from build123d import *

# Parameters (mm, degrees)
CROQUIS1_R              = 1.5
SALIENTE_EXTRUIR1_DEPTH = 1
CORTAR_EXTRUIR1_DEPTH   = 1


with BuildPart() as part:
    # Croquis1 → Saliente-Extruir1 (new body)
    with BuildSketch(Plane(origin=(0, 0, 0), x_dir=(1, 0, 0), z_dir=(0, 1, 0))):
        Polygon((-3, 3), (-3, -49.8), (3, -49.8), (3, -43.8), (29, -26.4), (35, -26.4), (35, -20.4), (29, -20.4), (3, -3), (3, 3), align=None)
        with Locations(Location((0, 0, 0), (0, 0, 270))):
            Circle(CROQUIS1_R, mode=Mode.SUBTRACT)
        with Locations(Location((0, -46.8, 0), (0, 0, 270))):
            Circle(CROQUIS1_R, mode=Mode.SUBTRACT)
        with Locations(Location((32, -23.4, 0), (0, 0, 270))):
            Circle(CROQUIS1_R, mode=Mode.SUBTRACT)
    extrude(amount=SALIENTE_EXTRUIR1_DEPTH)

    # Croquis2 → Cortar-Extruir1 (cut)
    with BuildSketch(Plane(origin=(0, 4, 0), x_dir=(1, 0, 0), z_dir=(0, 1, 0))):
        Polygon((29, -20.4), (29, -26.4), (1.37887203, -65.195749652), (-23.269516781, -18.416533666), (-7.63010581, 16.328115394), align=None)
    extrude(amount=-CORTAR_EXTRUIR1_DEPTH, mode=Mode.SUBTRACT)


solid = part.part
Part model, mm, in its own coordinate system. A direction names the side the tool comes from. Coordinates: 2 decimals unless noted, no trailing zeros. Order: outer loops, then holes, each group sorted by start corner. A loop starts at its lowest first (then second) coordinate and runs counter-clockwise, first axis right, second up. Notation, with made-up numbers: M 8,86 L 12,86 A12 ccw 12,104 Z; hole C 68,73 d7. An arc over 180 degrees is marked long. One line per question, with ' | ' between items.
Q1. 3-axis set-ups, long thin cutter, end or side, ignore diameter. For faces 4 (the face through (0.45, 0.49, 1.43)), 5 (the face through (3, 0.5, 46.8)), 6 (the face through (32, 0.5, 20.4)): which of +Z, -Z, +X, -X, +Y, -Y reach the whole face in a straight line?
A:
face 4: +Y, -Y | face 5: +Z, +X, +Y, -Y | face 6: -Z, +X, +Y, -Y
Q2. Pin check, flat tip, straight feed: P1, Ø0.5, axis at x = 31, y = 0.5, coming from the +Z side. Stop position of the tip, or through.
A:
P1: stops at z = 26.4
Q3. Drill centre lines: line 1 (Z direction, x = 1, y = 0.6); line 2 (X direction, y = 0.7, z = 46.8); line 3 (X direction, y = 0.25, z = 23.4). Where is each one in solid material? Low to high.
A:
line 1: z = -3 to -1.12, 1.12 to 45.68, 47.92 to 49.8 | line 2: x = -3 to -1.5, 1.5 to 3 | line 3: x = -3 to 30.5, 33.5 to 35
Q4. Slice it at C-C (x = 0). Give the cut face in (y, z), and give its area (3 significant figures).
A:
outline: M 0,-3 L 1,-3 L 1,-1.5 L 0,-1.5 Z; M 0,1.5 L 1,1.5 L 1,45.3 L 0,45.3 Z; M 0,48.3 L 1,48.3 L 1,49.8 L 0,49.8 Z | area: 46.8 mm^2
Q5. Slice it at D-D (y = 0.45). Give the cut face in (x, z), and give its area (3 significant figures).
A:
outline: M -3,-3 L 3,-3 L 3,3 L 29,20.4 L 35,20.4 L 35,26.4 L 29,26.4 L 3,43.8 L 3,49.8 L -3,49.8 Z; hole C 0,0 d3; hole C 0,46.8 d3; hole C 32,23.4 d3 | area: 940 mm^2
Q6. Slice it at A-A (z = 23.4). Give the cut face in (x, y).
A:
outline: M -3,0 L 30.5,0 L 30.5,1 L -3,1 Z; M 33.5,0 L 35,0 L 35,1 L 33.5,1 Z
Q7. Slice it at B-B (x = 32). Give the cut face in (y, z), and give its area (3 significant figures).
A:
outline: M 0,20.4 L 1,20.4 L 1,21.9 L 0,21.9 Z; M 0,24.9 L 1,24.9 L 1,26.4 L 0,26.4 Z | area: 3.00 mm^2
Q8. Two-plate mould, pull along Z, no slides. Class faces 1 (the face through (-3, 0.5, 23)), 2 (the face through (32, 0.5, 26.4)), 3 (the face through (31.425, 0.493, 24.786)): +Z half, -Z half, draft (parallel to the pull), parting line (faces both ways), or undercut.
A:
face 1: draft | face 2: +Z half | face 3: undercut
